from build123d import *

# Parameters (mm, degrees)
CHANFREIN1_SIZE         = 1
CONG_1_R                = 0.5
CHANFREIN2_SIZE         = 0.5
ENL_V_MAT_EXTRU_1_DEPTH = 15
CHANFREIN3_SIZE         = 0.5
ESQUISSE3_R             = 2
ENL_V_MAT_EXTRU_2_DEPTH = 96.372952141


with BuildPart() as part:
    # Esquisse1 → Base-Révolution (revolve)
    with BuildSketch(Plane.XY, mode=Mode.PRIVATE) as base_r_volution_sk:
        Polygon((0, 4.5), (0, 6), (-13, 6), (-13, 9.5), (-18, 9.5), (-20, 7.5), (-28, 7.5), (-28, 8), (-28.5, 8.5), (-35, 8.5), (-35, 11), (-61, 11), (-61, 14), (-74, 14), (-74, 11.5), (-88, 11.5), (-88, 8.5), (-76, 8.5), (-76, 6), (-66, 6), (-66, 4.5), align=None)
    revolve(base_r_volution_sk.sketch.rotate(Axis((11, 0, 0), (-1, 0, 0)), 90), axis=Axis((11, 0, 0), (-1, 0, 0)))

    # Chanfrein1
    chanfrein1_edges = [part.edges().sort_by_distance(p)[0] for p in [
        (-61, 0, 14),
        (-74, 0, 14),
        (-88, 0, 11.5),
    ]]
    chamfer(chanfrein1_edges, length=CHANFREIN1_SIZE)

    # Congé1
    cong_1_edges = [part.edges().sort_by_distance(p)[0] for p in [
        (-61, 0, 11),
    ]]
    fillet(cong_1_edges, radius=CONG_1_R)

    # Chanfrein2
    chanfrein2_edges = [part.edges().sort_by_distance(p)[0] for p in [
        (-88, 0, 8.5),
        (-76, 0, 6),
        (0, 0, 6),
        (-66, 0, 4.5),
    ]]
    chamfer(chanfrein2_edges, length=CHANFREIN2_SIZE)

    # Esquisse2 → Enlèv. mat.-Extru.1 (cut)
    with BuildSketch(Plane(origin=(-13, 0, 0), x_dir=(0, 0, -1), z_dir=(1, 0, 0))):
        Polygon((-7, 0), (-6.5, 9), (-14, 9), (-14, -9), (-6.5, -9), align=None)
        Polygon((14, -9), (6.5, -9), (7, 0), (6.5, 9), (14, 9), align=None)
    extrude(amount=-ENL_V_MAT_EXTRU_1_DEPTH, mode=Mode.SUBTRACT)

    # Chanfrein3
    chanfrein3_edges = [part.edges().sort_by_distance(p)[0] for p in [
        (-13, 9.5, 0),
        (-13, -9.5, 0),
    ]]
    chamfer(chanfrein3_edges, length=CHANFREIN3_SIZE)

    # Esquisse3 → Enlèv. mat.-Extru.2 (cut, through all)
    with BuildSketch(Plane.XY.offset(20)):
        with Locations((-82, 0)):
            Circle(ESQUISSE3_R)
    extrude(amount=-ENL_V_MAT_EXTRU_2_DEPTH, mode=Mode.SUBTRACT)


solid = part.part
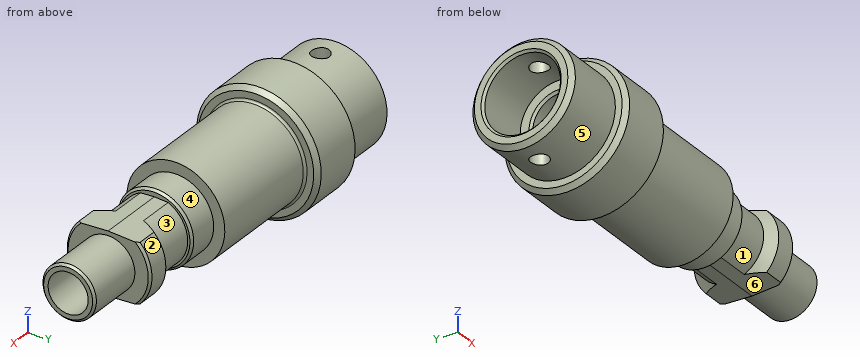
For this review, take the finished solid that the model builds, in its own axes (mm). Face numbers are marked on the shaded views. A direction names the side the tool comes from. Coordinates: 2 decimals unless noted, no trailing zeros. Order: outer loops, then holes, each group sorted by start corner. A loop starts at its lowest first (then second) coordinate and runs counter-clockwise, first axis right, second up. Notation, with made-up numbers: (-5.5, 5.5) - (44.5, 5.5) arc R11 ccw to (44.5, 23.5) - close; hole circle Ø4 at (29.25, -14). An arc over 180 degrees is marked (long way). Answer as CSV lines item,"result". Start each with the question number.
1) Add section A-A (x = -17). State the section outline as (y, z) points, then the cut area to 3 significant figures.
2) Machinability: for the marked faces 3, 4, 5 and 6, which of the approach directions +Z, -Z, +X, -X, +Y, -Y give a long, thin tool a straight path to every point of the face, cutting with its end or side? Answer none if there is none.
3) Draft analysis for pull direction X (two halves, no side actions). For the marked faces 1 and 2, state which applies: +X half, -X half, draft (parallel to the pull), parting line (faces both ways), or undercut.
4) To check wall thickness, follow line 1 along Y through (x, z) = (-71, 0); line 2 along Y through (x, z) = (-82, -9.4); line 3 along X through (y, z) = (10, 0.5). State the ranges of each line that lie inside material, in increasing order. Write a range as [from, to].
5) Insertion check: P1, Ø1.5, axis at x = -12, z = -3.5, coming from the +Y side; P2, Ø9.5, axis at y = 0, z = 0, coming from the -X side; P3, Ø1.5, axis at x = -30.5, z = 2.5, coming from the +Y side. Each pin has a flat end and moves straight along its axis. Give the tip position at first contact, or say it passes through.
6) Add section C-C (x = -51.5). State the section outline as (y, z) points, then the cut area to 3 significant figures.
7) Add section D-D (x = -31.5). State the section outline as (y, z) points.
8) Add section B-B (x = -82). State the section outline as (y, z) points, then the cut area to 3 significant figures.
Result:
1,outline,"(-6.81, -6.62) - (0, -7) - (6.81, -6.62) arc R9.5 ccw to (6.81, 6.62) - (0, 7) - (-6.81, 6.62) arc R9.5 ccw to start; hole circle Ø9 at (0, 0)"
1,area,"171 mm^2"
2,face 3,"+Y"
2,face 4,"none"
2,face 5,"-X"
2,face 6,"-Z, +X, -Y"
3,face 1,"undercut"
3,face 2,"draft"
4,line 1,"[-14, -6], [6, 14]"
4,line 2,"[-6.62, -2], [2, 6.62]"
4,line 3,"[-88, -35]"
5,P1,"y = 5.33"
5,P2,"x = -65.75"
5,P3,"y = 8.32"
6,outline,"circle Ø22 at (0, 0); hole circle Ø9 at (0, 0)"
6,area,"317 mm^2"
7,outline,"circle Ø17 at (0, 0); hole circle Ø9 at (0, 0)"
8,outline,"(-2, -11.32) - (-2, -8.26) arc R8.5 cw to (-2, 8.26) - (-2, 11.32) arc R11.5 ccw to start; (2, -11.32) arc R11.5 ccw to (2, 11.32) - (2, 8.26) arc R8.5 cw to (2, -8.26) - close"
8,area,"164 mm^2"
